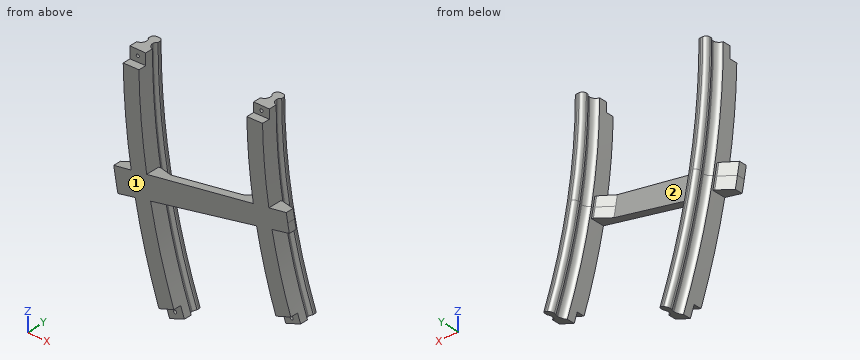
from build123d import *

# Parameters (mm, degrees)
REVOLVE_1_ANGLE     = 10
FILLET_1_R          = 1.5
FILLET_2_R          = 1.5
FILLET_3_R          = 1
FILLET_4_R          = 1
SKETCH_7_W          = 4
SKETCH_7_H          = 2
CUT_REVOLVE_1_ANGLE = 1
SKETCH_10_R         = 0.4
CUT_EXTRUDE_1_DEPTH = 2
REVOLVE_2_ANGLE     = 1


with BuildPart() as part:
    # 草图4 → 旋转1 (revolve)
    with BuildSketch(Plane.XY):
        Polygon((0.75, -1.5), (1.25, -1.5), (1.25, 0), (0, 0), (-1.25, 0), (-1.25, -1.5), (-0.75, -1.5), (-0.75, -4), (-2, -4), (-2, -8), (0, -8), (2, -8), (2, -4), (0.75, -4), align=None)
        Polygon((31.5, 0), (32.75, 0), (32.75, -1.5), (32.25, -1.5), (32.25, -4), (33.5, -4), (33.5, -8), (31.5, -8), (29.5, -8), (29.5, -4), (30.75, -4), (30.75, -1.5), (30.25, -1.5), (30.25, 0), align=None)
    revolve(axis=Axis((165.75, 3.853460973, 0), (0, -1, 0)), revolution_arc=REVOLVE_1_ANGLE)

    # 圆角1
    # the kernel refuses this fillet: 1.5 mm, written as the material it adds along each edge
    with BuildSketch(Plane(origin=(165.75, -4, 0), x_dir=(-1, 0, 0), z_dir=(0, 0, 1))) as fillet_1_piece_1:
        with BuildLine():
            CenterArc((163.5, -1.479019946), FILLET_1_R, 0, 80.405931773)
            Line((165, -1.479019946), (165.03, -1.479019946))
            Line((165.03, -1.479019946), (165.03, 0))
            Line((165.03, 0), (165, 0.03))
            ThreePointArc((165, 0.03), (164.375, 0.03), (163.755, 0.029580399))
            Line((163.755, 0.029580399), (163.75, 0))
        make_face()
    revolve(axis=Axis((165.75, -4, 0), (0, -1, 0)), revolution_arc=10)
    with BuildSketch(Plane(origin=(165.75, -4, 0), x_dir=(-1, 0, 0), z_dir=(0, 0, 1))) as fillet_1_piece_2:
        with BuildLine():
            CenterArc((168, -1.479019946), FILLET_1_R, 99.594068227, 80.405931773)
            Line((166.5, -1.479019946), (166.47, -1.479019946))
            Line((166.47, -1.479019946), (166.47, 0))
            Line((166.47, 0), (166.5, 0.03))
            ThreePointArc((166.5, 0.03), (167.125, 0.03), (167.745, 0.029580399))
            Line((167.745, 0.029580399), (167.75, 0))
        make_face()
    revolve(axis=Axis((165.75, -4, 0), (0, -1, 0)), revolution_arc=10)

    # 圆角2
    # the kernel refuses this fillet: 1.5 mm, written as the material it adds along each edge
    with BuildSketch(Plane(origin=(165.75, -4, 0), x_dir=(-1, 0, 0), z_dir=(0, 0, 1))) as fillet_2_piece_1:
        with BuildLine():
            CenterArc((136.5, -1.479019946), FILLET_2_R, 99.594068227, 80.405931773)
            Line((136.25, 0), (136.245, 0.029580399))
            ThreePointArc((136.245, 0.029580399), (135.625, 0.03), (135, 0.03))
            Line((135, 0.03), (134.97, 0))
            Line((134.97, 0), (134.97, -1.479019946))
            Line((134.97, -1.479019946), (135, -1.479019946))
        make_face()
    revolve(axis=Axis((165.75, -4, 0), (0, -1, 0)), revolution_arc=10)
    with BuildSketch(Plane(origin=(165.75, -4, 0), x_dir=(-1, 0, 0), z_dir=(0, 0, 1))) as fillet_2_piece_2:
        with BuildLine():
            CenterArc((132, -1.479019946), FILLET_2_R, 0, 80.405931773)
            Line((133.5, -1.479019946), (133.53, -1.479019946))
            Line((133.53, -1.479019946), (133.53, 0))
            Line((133.53, 0), (133.5, 0.03))
            ThreePointArc((133.5, 0.03), (132.875, 0.03), (132.255, 0.029580399))
            Line((132.255, 0.029580399), (132.25, 0))
        make_face()
    revolve(axis=Axis((165.75, -4, 0), (0, -1, 0)), revolution_arc=10)

    # 圆角3
    # the kernel refuses this fillet: 1 mm, written as the material it adds along each edge
    with BuildSketch(Plane(origin=(165.75, -1.5, 0), x_dir=(-1, 0, 0), z_dir=(0, 0, 1))) as fillet_3_piece_1:
        with BuildLine():
            CenterArc((136, 0.866025404), FILLET_3_R, 180, 60)
            Line((135, 0.866025404), (135, 0))
            Line((135, 0), (135.5, 0))
        make_face()
    revolve(axis=Axis((165.75, -1.5, 0), (0, -1, 0)), revolution_arc=10)
    with BuildSketch(Plane(origin=(165.75, -1.5, 0), x_dir=(-1, 0, 0), z_dir=(0, 0, 1))) as fillet_3_piece_2:
        with BuildLine():
            CenterArc((132.5, 0.866025404), FILLET_3_R, 300, 60)
            Line((133, 0), (133.5, 0))
            Line((133.5, 0), (133.5, 0.866025404))
        make_face()
    revolve(axis=Axis((165.75, -1.5, 0), (0, -1, 0)), revolution_arc=10)
    # the kernel refuses this fillet: 1 mm, written as the material it takes off along each edge
    with BuildSketch(Plane(origin=(165.75, 0, 0), x_dir=(-0.9998233399867428, 0, 0.018795978765534377), z_dir=(0.018795978765534377, 0, 0.9998233399867428))) as fillet_3_2_piece_1:
        with BuildLine():
            CenterArc((133 + FILLET_3_R, FILLET_3_R), FILLET_3_R, 180, 90)
            Line((133, FILLET_3_R), (133, 0))
            Line((133, 0), (133 + FILLET_3_R, 0))
        make_face()
    revolve(axis=Axis((165.75, 0, 0), (0, -1, 0)), revolution_arc=12.153987353, mode=Mode.SUBTRACT)
    with BuildSketch(Plane(origin=(165.75, 0, 0), x_dir=(-0.9998297984864879, 0, 0.01844922921070363), z_dir=(0.01844922921070363, 0, 0.9998297984864879))) as fillet_3_2_piece_2:
        with BuildLine():
            CenterArc((135.5 - FILLET_3_R, FILLET_3_R), FILLET_3_R, 270, 90)
            Line((135.5 - FILLET_3_R, 0), (135.5, 0))
            Line((135.5, 0), (135.5, FILLET_3_R))
        make_face()
    revolve(axis=Axis((165.75, 0, 0), (0, -1, 0)), revolution_arc=12.114245889, mode=Mode.SUBTRACT)

    # 圆角4
    # the kernel refuses this fillet: 1 mm, written as the material it adds along each edge
    with BuildSketch(Plane(origin=(165.75, -1.5, 0), x_dir=(-1, 0, 0), z_dir=(0, 0, 1))) as fillet_4_piece_1:
        with BuildLine():
            CenterArc((167.5, 0.866025404), FILLET_4_R, 180, 60)
            Line((167, 0), (166.5, 0))
            Line((166.5, 0), (166.5, 0.866025404))
        make_face()
    revolve(axis=Axis((165.75, -1.5, 0), (0, -1, 0)), revolution_arc=10)
    with BuildSketch(Plane(origin=(165.75, -1.5, 0), x_dir=(-1, 0, 0), z_dir=(0, 0, 1))) as fillet_4_piece_2:
        with BuildLine():
            CenterArc((164, 0.866025404), FILLET_4_R, 300, 60)
            Line((164.5, 0), (165, 0))
            Line((165, 0), (165, 0.866025404))
        make_face()
    revolve(axis=Axis((165.75, -1.5, 0), (0, -1, 0)), revolution_arc=10)
    # the kernel refuses this fillet: 1 mm, written as the material it takes off along each edge
    with BuildSketch(Plane(origin=(165.75, 0, 0), x_dir=(-0.9998845180351503, 0, 0.015197058715919934), z_dir=(0.015197058715919934, 0, 0.9998845180351503))) as fillet_4_2_piece_1:
        with BuildLine():
            CenterArc((164.5 + FILLET_4_R, FILLET_4_R), FILLET_4_R, 180, 90)
            Line((164.5, FILLET_4_R), (164.5, 0))
            Line((164.5, 0), (164.5 + FILLET_4_R, 0))
        make_face()
    revolve(axis=Axis((165.75, 0, 0), (0, -1, 0)), revolution_arc=11.74152169, mode=Mode.SUBTRACT)
    with BuildSketch(Plane(origin=(165.75, 0, 0), x_dir=(-0.9998879496351009, 0, 0.014969574961036002), z_dir=(0.014969574961036002, 0, 0.9998879496351009))) as fillet_4_2_piece_2:
        with BuildLine():
            CenterArc((167 - FILLET_4_R, FILLET_4_R), FILLET_4_R, 270, 90)
            Line((167 - FILLET_4_R, 0), (167, 0))
            Line((167, 0), (167, FILLET_4_R))
        make_face()
    revolve(axis=Axis((165.75, 0, 0), (0, -1, 0)), revolution_arc=11.715451006, mode=Mode.SUBTRACT)

    # 草图7 → 切除-旋转1 (revolve, cut)
    with BuildSketch(Plane.XY):
        with Locations((0, -7)):
            Rectangle(SKETCH_7_W, SKETCH_7_H)
        with Locations((31.5, -7)):
            Rectangle(SKETCH_7_W, SKETCH_7_H)
    revolve(axis=Axis((165.75, 3.853460973, 0), (0, -1, 0)), revolution_arc=CUT_REVOLVE_1_ANGLE, mode=Mode.SUBTRACT)

    # 草图10 → 切除-拉伸1 (cut)
    with BuildSketch(Plane.XZ.offset(6)):
        with Locations(Location((0.006311252, -1.446423259, 0), (0, 0, 270))):
            Circle(SKETCH_10_R)
        with Locations(Location((31.505111829, -1.171537391, 0), (0, 0, 270))):
            Circle(SKETCH_10_R)
    extrude(amount=-CUT_EXTRUDE_1_DEPTH, mode=Mode.SUBTRACT)

    # 草图11 → 旋转2 (revolve)
    with BuildSketch(Plane(origin=(4.997974052, 0, -28.344919378), x_dir=(-0.9848077530122081, 0, -0.17364817766693072), z_dir=(0.17364817766693072, 0, -0.9848077530122081))):
        Polygon((-26.981885062, -4.5), (-26.481885062, -4.5), (-22.481885062, -6), (-3.981885062, -6), (0.018114938, -4.5), (0.518114938, -4.5), (4.518114938, -4.5), (5.018114938, -4.5), (9.018114938, -6), (9.018114938, -8), (4.518114938, -8), (0.518114938, -8), (-26.981885062, -8), (-30.981885062, -8), (-35.481885062, -8), (-35.481885062, -6), (-31.481885062, -4.5), (-30.981885062, -4.5), align=None)
    revolve(axis=Axis((165.75, 3.853460973, 0), (0, 1, 0)), revolution_arc=REVOLVE_2_ANGLE)

    # 镜向1: part across face


with BuildPart() as part_1:
    add(part.part)
    add(part.part.mirror(Plane(origin=(18.028837048, -5.996688627, -26.04722665), x_dir=(0.9848077529548817, 0, 0.17364817799204443), z_dir=(0.17364817799204443, 0, -0.9848077529548818))))


solid = part_1.part
CAD build for the part. Positions are in the model's coordinates, mm. Face numbers are marked on the shaded views. Give positions to 0.01 mm unless a question says otherwise; leave off trailing zeros. Write each loop counter-clockwise with the first axis right and the second up, starting at its lowest first coordinate (ties: lowest second). Pieces come first, ordered by that corner, then holes. Notation, with made-up numbers: M 1,67.5 L 26,67.5 A18 cw 26,91.5 Z; hole C 14.5,-28.5 d9. An arc over 180 degrees is marked long. Put each result on its own line as item: value. Start each with the question number.
(1) Band-saw the part on C-C, the plane x = 23. Write the cut outline in (y, z), and give its area (3 significant figures).
(2) Flat gauge pins, fed straight in: pin 1 Ø8 at (x, z) = (12.5, -36) entering from -Y; pin 2 Ø0.6 at (x, z) = (36, -23) entering from +Y; pin 3 Ø0.9 at (x, z) = (31.5, -1) entering from -Y; pin 4 Ø1.6 at (x, z) = (5, -27.5) entering from +Y. Where does each tip first touch, or does it go through?
(3) Probe L1, parallel to Y at x = 18.5, z = -24; L2, parallel to X at y = -5.5, z = -10; L3, parallel to X at y = -3.75, z = -34.5. List the from-to ranges inside material, lowest first.
(4) Band-saw the part on B-B, the plane y = -7. Write the cut outline in (x, z).
(5) Mould opens along X. For the marked faces 1 and 2 say: +X half, -X half, draft (parallel to the pull), parting line (faces both ways), or undercut.
(6) Band-saw the part on A-A, the plane y = -3.25. Write the cut outline in (x, z), and give its area (3 significant figures).
Response values:
1. outline: M -8,-27.75 L -6,-27.75 L -6,-22.61 L -8,-22.61 Z
1. area: 10.3 mm2
2. pin 1: passes through
2. pin 2: stops at y = -4.5
2. pin 3: stops at y = -6
2. pin 4: stops at y = -3.97
3. L1: y = -8 to -6
3. L2: x = -1.7 to 2.31, 29.87 to 33.88
3. L3: x = 2.21 to 5.05, 34.57 to 37.45
4. outline: M -4.38,-26.95 A172.25 ccw -3.34,-32.87 L 1.08,-32.01 A167.75 ccw 7.14,-54.61 L 10.92,-53.31 A163.75 cw 5.01,-31.24 L 32,-26 A136.25 ccw 36.92,-44.36 L 40.71,-43.06 A132.25 cw 35.93,-25.23 L 40.35,-24.38 A127.75 cw 39.57,-19.98 L 35.13,-20.69 A132.25 cw 33.52,-2.31 L 29.52,-2.38 A136.25 ccw 31.18,-21.31 L 4.02,-25.62 A163.75 cw 2.02,-2.86 L -1.97,-2.93 A167.75 ccw 0.07,-26.24 Z
5. face 1: draft
5. face 2: undercut
6. outline: M -0.94,0 A166.69 ccw 9.11,-57.01 L 10.88,-56.37 A164.81 cw 0.94,0 Z; M 30.56,0 A135.19 ccw 38.71,-46.24 L 40.48,-45.6 A133.31 cw 32.44,0 Z
6. area: 197 mm2
